Geometry: final body of the model. Coordinates: model frame, mm. Face numbers are marked on the shaded views. A direction names the side the tool comes from. Round coordinates to 2 decimals unless told otherwise and drop trailing zeros. Loops run counter-clockwise (first coordinate to the right, second up) from the corner with the lowest first, then second, coordinate; pieces in that order, holes last. Notation, with made-up numbers: M 39,-33.5 L 71,-33.5 A7 ccw 71,-28.5 Z; hole C 74,11.25 d6. An arc over 180 degrees is marked long. Return JSON: item names as keys, results as strings.
Autodesk Inventor part; units mm, degrees
ref_plane "YZ Plane" through (0, 0, 0) normal (1, 0, 0) x (0, 1, 0)
ref_plane "XZ Plane" through (0, 0, 0) normal (0, 1, 0) x (-1, 0, 0)
ref_plane "XY Plane" through (0, 0, 0) normal (0, 0, 1) x (1, 0, 0)
sketch "Sketch1" plane through (0, 0, 0) normal (0, 0, 1) x (1, 0, 0)
  line L0 (0, 0) -> (114.3, 0)
  line L1 (114.3, 0) -> (114.3, 25.4)
  line L2 (114.3, 25.4) -> (0, 25.4)
  line L3 (0, 25.4) -> (0, 0)
  dimension "d0" = 114.3
  dimension "d1" = 25.4
extrude "Extrusion1" add sketch "Sketch1" along normal blind 3.175
sketch "Sketch2" plane through (0, 0, 3.175) normal (0, 0, 1) x (1, 0, 0)
  line L0 (0, 0) -> (114.3, 0)
  line L1 (0, 0) -> (114.3, 0)
  line L2 (114.3, 0) -> (114.3, 3.175)
  line L3 (114.3, 0) -> (114.3, 25.4)
  line L4 (114.3, 3.175) -> (0, 3.175)
  line L5 (0, 3.175) -> (0, 0)
  dimension "d4" = 3.175
extrude "Extrusion2" add sketch "Sketch2" along normal blind 22.225
sketch "Sketch3" plane through (0, 0, 0) normal (0, -1, 0) x (1, 0, 0)
  line L0 (0, 0) -> (0, 25.4)
  line L1 (114.3, 0) -> (114.3, 25.4)
  line L2 (0, 0) -> (114.3, 0)
  point P0 (12.7, 14.605)
  point P1 (38.1, 14.605)
  point P2 (50.8, 14.605)
  point P3 (63.5, 14.605)
  point P4 (76.2, 14.605)
  point P5 (88.9, 14.605)
  point P6 (101.6, 14.605)
  point P7 (25.4, 14.605)
  dimension "d7" = 12.7
  dimension "d9" = 12.7
  dimension "d10" = 12.7
  dimension "d11" = 12.7
  dimension "d12" = 12.7
  dimension "d13" = 12.7
  dimension "d14" = 12.7
  dimension "d15" = 14.605
  dimension "d16" = 14.605
  dimension "d17" = 14.605
  dimension "d18" = 14.605
  dimension "d19" = 14.605
  dimension "d20" = 14.605
  dimension "d21" = 14.605
  dimension "d29" = 12.7
  dimension "d30" = 14.605
hole "Hole1" at (12.7, 0, 14.605) at (38.1, 0, 14.605) at (50.8, 0, 14.605) at (63.5, 0, 14.605) at (76.2, 0, 14.605) at (88.9, 0, 14.605) at (101.6, 0, 14.605) at (25.4, 0, 14.605) direction (0, 1, 0) diameter 6.731 depth 25.4 tip angle 118
properties part number "4 L aluminum piece for transmission bracket"
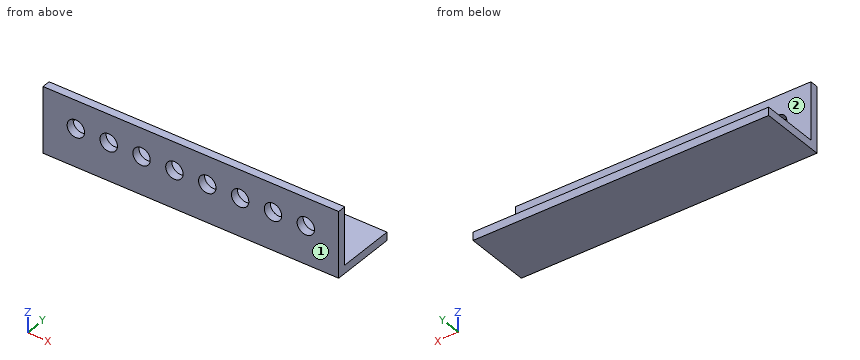
Q1. Section query C-C (z = 7.5). Output: boundary loops of the cut face in (x, y) (3 decimals), plus the area to 3 significant figures.
Determined:
{"outline": "M 0,0 L 114.3,0 L 114.3,3.175 L 0,3.175 Z", "area": "363 mm^2"}
Q2. Pin query (flat end, axial travel): pin 1 (9 mm diameter, centred on x = 25.4, z = 14.605, fed in from +Y) (3 decimals); pin 2 (1.5 mm diameter, centred on x = 21, y = 11.5, fed in from +Z) (3 decimals). Return the tip coordinate at first contact, or that it passes through.
Determined:
{"pin 1": "stops at y = 3.175", "pin 2": "stops at z = 3.175"}
Q3. Section query D-D (x = 69.5). Output: boundary loops of the cut face in (y, z) (3 decimals), plus the area to 3 significant figures.
Determined:
{"outline": "M 0,0 L 25.4,0 L 25.4,3.175 L 3.175,3.175 L 3.175,25.4 L 0,25.4 Z", "area": "151 mm^2"}
Q4. Material intervals for L1, parallel to Z at x = 76.2, y = 0.9; L2, parallel to Z at x = 33, y = 3.25 (3 decimals), sorted ascending.
Determined:
{"L1": "z = 0 to 11.24, 17.97 to 25.4", "L2": "z = 0 to 3.175"}
Q5. Section query A-A (x = 88.9). Output: boundary loops of the cut face in (y, z) (1 decimal), plus the area to 3 significant figures.
Determined:
{"outline": "M 0,0 L 25.4,0 L 25.4,3.2 L 3.2,3.2 L 3.2,11.2 L 0,11.2 Z; M 0,18 L 3.2,18 L 3.2,25.4 L 0,25.4 Z", "area": "130 mm^2"}
Q6. Section query B-B (y = 2). State how many separate pieces and enclosed holes the cut face has, plus the area to 3 significant figures.
Determined:
{"separate pieces": "1", "enclosed holes": "8", "area": "2,620 mm^2"}
Q7. Reachability of the marked faces 1 and 2 from +Z, -Z, +X, -X, +Y, -Y: full face, straight path, thin tool, end or side. Return the list, or none.
Determined:
{"face 1": "+Z, -Z, +X, -X, -Y", "face 2": "+Z, +X, -X, +Y"}
